from build123d import *

# Parameters (mm, degrees)
F1_DEPTH = 12.7
F2_R     = 4.445
F3_SIZE  = 1.5875


with BuildPart() as f1:
    # F0 (on Top) → F1 (new body, symmetric)
    with BuildSketch(Plane.XY):
        with BuildLine():
            ThreePointArc((26.209303, 32.602941), (24.094546, 36.53219), (19.916848, 38.1))
            Line((19.916848, 38.1), (-19.973807, 38.1))
            ThreePointArc((-19.973807, 38.1), (-24.128411, 36.552266), (-26.257749, 32.663547))
            ThreePointArc((-26.257749, 32.663547), (-28.619616, 0), (-26.257749, -32.663547))
            ThreePointArc((-26.257749, -32.663547), (-24.128411, -36.552266), (-19.973807, -38.1))
            Line((-19.973807, -38.1), (19.916848, -38.1))
            ThreePointArc((19.916848, -38.1), (24.094546, -36.53219), (26.209303, -32.602941))
            ThreePointArc((26.209303, -32.602941), (28.408907, 0), (26.209303, 32.602941))
        make_face()
        with BuildLine():
            ThreePointArc((-20.176107, -30.325869), (-21.360101, -20.015452), (-22.058065, -9.660772))
            ThreePointArc((-22.058065, -9.660772), (-21.601359, -8.446905), (-20.408647, -7.9375))
            Line((-20.408647, -7.9375), (-13.081, -7.9375))
            ThreePointArc((-13.081, -7.9375), (-11.913567, -8.421067), (-11.43, -9.5885))
            Line((-11.43, -9.5885), (-11.43, -30.099001))
            ThreePointArc((-11.43, -30.099001), (-11.913567, -31.266434), (-13.081, -31.750001))
            Line((-13.081, -31.750001), (-18.540769, -31.750001))
            ThreePointArc((-18.540769, -31.750001), (-19.625029, -31.344063), (-20.176107, -30.325869))
        make_face(mode=Mode.SUBTRACT)
        with BuildLine():
            ThreePointArc((20.107444, -30.310712), (19.56009, -31.339028), (18.470075, -31.750001))
            Line((18.470075, -31.750001), (13.081, -31.750001))
            ThreePointArc((13.081, -31.750001), (11.913567, -31.266434), (11.43, -30.099001))
            Line((11.43, -30.099001), (11.43, -9.5885))
            ThreePointArc((11.43, -9.5885), (11.913567, -8.421067), (13.081, -7.9375))
            Line((13.081, -7.9375), (20.211979, -7.9375))
            ThreePointArc((20.211979, -7.9375), (21.403018, -8.44516), (21.861601, -9.655944))
            ThreePointArc((21.861601, -9.655944), (21.21105, -20.002567), (20.107444, -30.310712))
        make_face(mode=Mode.SUBTRACT)
        with BuildLine():
            ThreePointArc((-22.058065, 9.660772), (-21.360101, 20.015452), (-20.176107, 30.325868))
            ThreePointArc((-20.176107, 30.325868), (-19.625029, 31.344062), (-18.540769, 31.75))
            Line((-18.540769, 31.75), (-13.081, 31.75))
            ThreePointArc((-13.081, 31.75), (-11.913567, 31.266433), (-11.43, 30.099))
            Line((-11.43, 30.099), (-11.43, 9.5885))
            ThreePointArc((-11.43, 9.5885), (-11.913567, 8.421067), (-13.081, 7.9375))
            Line((-13.081, 7.9375), (-20.408647, 7.9375))
            ThreePointArc((-20.408647, 7.9375), (-21.601359, 8.446905), (-22.058065, 9.660772))
        make_face(mode=Mode.SUBTRACT)
        with BuildLine():
            Line((13.081, 31.75), (18.470075, 31.75))
            ThreePointArc((18.470075, 31.75), (19.56009, 31.339028), (20.107444, 30.310712))
            ThreePointArc((20.107444, 30.310712), (21.21105, 20.002566), (21.861601, 9.655944))
            ThreePointArc((21.861601, 9.655944), (21.403018, 8.44516), (20.211979, 7.9375))
            Line((20.211979, 7.9375), (13.081, 7.9375))
            ThreePointArc((13.081, 7.9375), (11.913567, 8.421067), (11.43, 9.5885))
            Line((11.43, 9.5885), (11.43, 30.099))
            ThreePointArc((11.43, 30.099), (11.913567, 31.266433), (13.081, 31.75))
        make_face(mode=Mode.SUBTRACT)
    extrude(amount=F1_DEPTH, both=True)

    # F2
    f2_edges = [f1.edges().sort_by_distance(p)[0] for p in [
        (11.43, -19.84375, 12.7),
        (-11.43, -19.84375, 12.7),
        (11.43, 19.84375, 12.7),
        (-11.43, 19.84375, 12.7),
    ]]
    fillet(f2_edges, radius=F2_R)

    # F3
    f3_edges = [f1.edges().sort_by_distance(p)[0] for p in [
        (-0.028479, -38.1, 12.7),
    ]]
    chamfer(f3_edges, length=F3_SIZE)


solid = f1.part
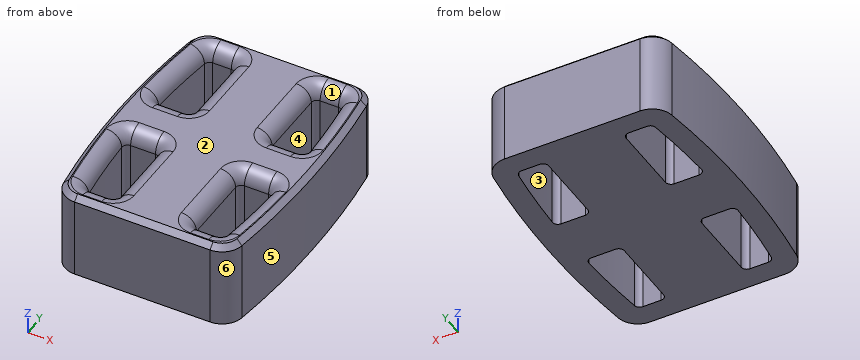
Source: CAD feature listing. Evaluate the final solid. Frame: model axes, mm. Face numbers are marked on the shaded views. A direction names the side the tool comes from. Give positions to 0.01 mm unless a question says otherwise; leave off trailing zeros. Use a Markdown table: item, result. Add a question column.
1) Line query: line 1 along Y through (x, z) = (15, 3.75); line 2 along X through (y, z) = (-12.5, -9); line 3 along Y through (x, z) = (-19, -3.5). Output: solid intervals per line, ascending. Write a range as [from, to].
2) First-contact query: pin 1 (10.5 mm diameter, centred on y = -23, z = 0, fed in from +X); pin 2 (2 mm diameter, centred on y = -23, z = -2, fed in from +X); pin 3 (10.5 mm diameter, centred on y = 22.5, z = 0, fed in from -X). Flat tips, straight axial feed; report the tip coordinate or a pass-through.
3) Reachability of the marked faces 1, 2 and 3 from +Z, -Z, +X, -X, +Y, -Y: full face, straight path, thin tool, end or side. Return the list, or none.
4) Pull-direction query (Y, two-part tool) for the marked faces 4, 5 and 6; classes: +Y half, -Y half, draft (parallel to the pull), parting line (faces both ways), or undercut.
5) Section query A-A, the plane x = 14. Count the separate pieces of the cut face and the enclosed holes in it, then the cut area to 3 significant figures.
Numbers:
| question | item | result |
|---|---|---|
| 1 | line 1 | y = [-38.1, -31.75], [-7.94, 7.94], [31.75, 38.1] |
| 1 | line 2 | x = [-28.28, -21.92], [-11.43, 11.43], [21.73, 28.09] |
| 1 | line 3 | y = [-38.1, -31.68], [-7.94, 7.94], [31.68, 38.1] |
| 2 | pin 1 | stops at x = 27.76 |
| 2 | pin 2 | stops at x = 27.41 |
| 2 | pin 3 | stops at x = -27.96 |
| 3 | face 1 | +Z |
| 3 | face 2 | +Z, +X, -X, +Y, -Y |
| 3 | face 3 | +Z, -Z |
| 4 | face 4 | undercut |
| 4 | face 5 | parting line |
| 4 | face 6 | -Y half |
| 5 | separate pieces | 3 |
| 5 | enclosed holes | 0 |
| 5 | area | 706 mm2 |
